```python
from build123d import *

# Parameters (mm, degrees)
AUFSATZ_LINEAR_AUSTRAGEN1_DEPTH      = 2.5
AUFSATZ_LINEAR_AUSTRAGEN1_DEPTH_BACK = 2.5
SKIZZE1_W                            = 100
SKIZZE1_H                            = 40
SCHNITT_LINEAR_AUSTRAGEN1_DEPTH      = 54.909646632
SCHNITT_LINEAR_AUSTRAGEN1_DEPTH_BACK = 54.909646632
SKIZZE2_R                            = 1.5
SCHNITT_LINEAR_AUSTRAGEN2_DEPTH      = 54.909646632
SCHNITT_LINEAR_AUSTRAGEN2_DEPTH_BACK = 54.909646632
SKIZZE7_W                            = 70
SKIZZE7_H                            = 40
AUFSATZ_LINEAR_AUSTRAGEN3_DEPTH      = 5
FASE1_SIZE                           = 2
SCHNITT_LINEAR_AUSTRAGEN7_DEPTH      = 55.371407927
SCHNITT_LINEAR_AUSTRAGEN7_DEPTH_BACK = 55.371407927
VERRUNDUNG1_R                        = 2
SCHNITT_LINEAR_AUSTRAGEN6_DEPTH      = 8.5
VERRUNDUNG2_R                        = 2
SCHNITT_LINEAR_AUSTRAGEN8_DEPTH      = 59.285933123
VERRUNDUNG3_R                        = 1
VERRUNDUNG4_R                        = 6


with BuildPart() as part:
    # Skizze1 → Aufsatz-Linear austragen1 (new, two sides: drawn at the far end of the back side and taken through both)
    with BuildSketch(Plane.XY.offset(-AUFSATZ_LINEAR_AUSTRAGEN1_DEPTH_BACK)):
        Rectangle(SKIZZE1_W, SKIZZE1_H)
    extrude(amount=AUFSATZ_LINEAR_AUSTRAGEN1_DEPTH + AUFSATZ_LINEAR_AUSTRAGEN1_DEPTH_BACK)

    # Skizze2 → Schnitt-Linear austragen1 (cut, two sides: drawn at the far end of the back side and taken through both)
    with BuildSketch(Plane.XY.offset(-SCHNITT_LINEAR_AUSTRAGEN1_DEPTH_BACK)):
        with Locations((-45, 15)):
            Circle(SKIZZE2_R)
        with Locations(Location((-45, -15, 0), (0, 0, 180))):
            Circle(SKIZZE2_R)
        with Locations((45, -15)):
            Circle(SKIZZE2_R)
        with Locations(Location((45, 15, 0), (0, 0, 180))):
            Circle(SKIZZE2_R)
    extrude(amount=SCHNITT_LINEAR_AUSTRAGEN1_DEPTH + SCHNITT_LINEAR_AUSTRAGEN1_DEPTH_BACK, mode=Mode.SUBTRACT)

    # Skizze4 → Schnitt-Linear austragen2 (cut, two sides: drawn at the far end of the back side and taken through both)
    with BuildSketch(Plane.XY.offset(-SCHNITT_LINEAR_AUSTRAGEN2_DEPTH_BACK)):
        with BuildLine():
            Line((-48, -8), (-48, 8))
            ThreePointArc((-48, 8), (-47.121320344, 10.121320344), (-45, 11))
            Line((-45, 11), (-40.5, 11))
            ThreePointArc((-40.5, 11), (-38.378679656, 10.121320344), (-37.5, 8))
            Line((-37.5, 8), (-37.5, -8))
            ThreePointArc((-37.5, -8), (-38.378679656, -10.121320344), (-40.5, -11))
            Line((-40.5, -11), (-45, -11))
            ThreePointArc((-45, -11), (-47.121320344, -10.121320344), (-48, -8))
        make_face()
        with BuildLine():
            Line((45, -11), (40.5, -11))
            ThreePointArc((40.5, -11), (38.378679656, -10.121320344), (37.5, -8))
            Line((37.5, -8), (37.5, 8))
            ThreePointArc((37.5, 8), (38.378679656, 10.121320344), (40.5, 11))
            Line((40.5, 11), (45, 11))
            ThreePointArc((45, 11), (47.121320344, 10.121320344), (48, 8))
            Line((48, 8), (48, -8))
            ThreePointArc((48, -8), (47.121320344, -10.121320344), (45, -11))
        make_face()
    extrude(amount=SCHNITT_LINEAR_AUSTRAGEN2_DEPTH + SCHNITT_LINEAR_AUSTRAGEN2_DEPTH_BACK, mode=Mode.SUBTRACT)

    # Skizze7 → Aufsatz-Linear austragen3 (add)
    with BuildSketch(Plane(origin=(0, 0, -2.5), x_dir=(-1, 0, 0), z_dir=(0, 0, -1))):
        Rectangle(SKIZZE7_W, SKIZZE7_H)
    extrude(amount=AUFSATZ_LINEAR_AUSTRAGEN3_DEPTH)

    # Fase1
    fase1_edges = [part.edges().sort_by_distance(p)[0] for p in [
        (50, 20, 0),
        (50, -20, 0),
        (-50, -20, 0),
        (-50, 20, 0),
    ]]
    chamfer(fase1_edges, length=FASE1_SIZE)

    # Skizze9 → Schnitt-Linear austragen7 (cut, two sides: drawn at the far end of the back side and taken through both)
    with BuildSketch(Plane.XY.offset(-SCHNITT_LINEAR_AUSTRAGEN7_DEPTH_BACK)):
        with BuildLine():
            Line((-3.5, -20), (3.5, -20))
            Line((3.5, -20), (3.5, -7))
            ThreePointArc((3.5, -7), (0, -3.5), (-3.5, -7))
            Line((-3.5, -7), (-3.5, -20))
        make_face()
    extrude(amount=SCHNITT_LINEAR_AUSTRAGEN7_DEPTH + SCHNITT_LINEAR_AUSTRAGEN7_DEPTH_BACK, mode=Mode.SUBTRACT)

    # Verrundung1
    verrundung1_edges = [part.edges().sort_by_distance(p)[0] for p in [
        (3.5, -20, -2.5),
        (-3.5, -20, -2.5),
    ]]
    fillet(verrundung1_edges, radius=VERRUNDUNG1_R)

    # Skizze8 → Schnitt-Linear austragen6 (cut)
    with BuildSketch(Plane.XY.offset(2.5)):
        with BuildLine():
            Line((6.5, -18), (30, -18))
            ThreePointArc((30, -18), (32.121320344, -17.121320344), (33, -15))
            Line((33, -15), (33, 15))
            ThreePointArc((33, 15), (32.121320344, 17.121320344), (30, 18))
            Line((30, 18), (-30, 18))
            ThreePointArc((-30, 18), (-32.121320344, 17.121320344), (-33, 15))
            Line((-33, 15), (-33, -15))
            ThreePointArc((-33, -15), (-32.121320344, -17.121320344), (-30, -18))
            Line((-30, -18), (-6.5, -18))
            ThreePointArc((-6.5, -18), (-5.792893219, -17.707106781), (-5.5, -17))
            Line((-5.5, -17), (-5.5, -7))
            ThreePointArc((-5.5, -7), (0, -1.5), (5.5, -7))
            Line((5.5, -7), (5.5, -17))
            ThreePointArc((5.5, -17), (5.792893219, -17.707106781), (6.5, -18))
        make_face()
    extrude(amount=-SCHNITT_LINEAR_AUSTRAGEN6_DEPTH, mode=Mode.SUBTRACT)

    # Verrundung2
    # the kernel refuses this fillet: 2 mm, written as the material it takes off along each edge
    with BuildSketch(Plane(origin=(-3.5, -7, -7.5), x_dir=(0, 0, 1), z_dir=(0, -1, 0)), Plane(origin=(3.5, -23, -7.5), x_dir=(0, 0, 1), z_dir=(0, 1, 0))) as verrundung2_piece_1:
        with BuildLine():
            CenterArc((VERRUNDUNG2_R, VERRUNDUNG2_R), VERRUNDUNG2_R, 180, 90)
            Line((0, VERRUNDUNG2_R), (0, 0))
            Line((0, 0), (VERRUNDUNG2_R, 0))
        make_face()
    extrude(amount=16, mode=Mode.SUBTRACT)
    with BuildSketch(Plane(origin=(0, -7, -7.5), x_dir=(-1, 0, 0), z_dir=(0, -1, 0))) as verrundung2_piece_2:
        with BuildLine():
            CenterArc((3.5 + VERRUNDUNG2_R, -VERRUNDUNG2_R), VERRUNDUNG2_R, 90, 90)
            Line((3.5 + VERRUNDUNG2_R, 0), (3.5, 0))
            Line((3.5, 0), (3.5, -VERRUNDUNG2_R))
        make_face()
    revolve(axis=Axis((0, -7, -7.5), (0, 0, -1)), revolution_arc=180, mode=Mode.SUBTRACT)

    # Skizze10 → Schnitt-Linear austragen8 (cut, through all)
    with BuildSketch(Plane(origin=(0, -9, 0), x_dir=(1, 0, 0), z_dir=(0, 1, 0))):
        Polygon((12, -2.5), (5.5, 4), (-5.5, 4), (-12, -2.5), align=None)
    extrude(amount=-SCHNITT_LINEAR_AUSTRAGEN8_DEPTH, mode=Mode.SUBTRACT)

    # Verrundung3
    verrundung3_edges = [part.edges().sort_by_distance(p)[0] for p in [
        (4.5, -9, 2.5),
        (4.5, -9, -4),
        (-4.5, -9, -4),
        (-4.5, -9, 2.5),
    ]]
    fillet(verrundung3_edges, radius=VERRUNDUNG3_R)

    # Verrundung4
    verrundung4_edges = [part.edges().sort_by_distance(p)[0] for p in [
        (12, -19, 2.5),
        (-12, -19, 2.5),
    ]]
    fillet(verrundung4_edges, radius=VERRUNDUNG4_R)


solid = part.part
```
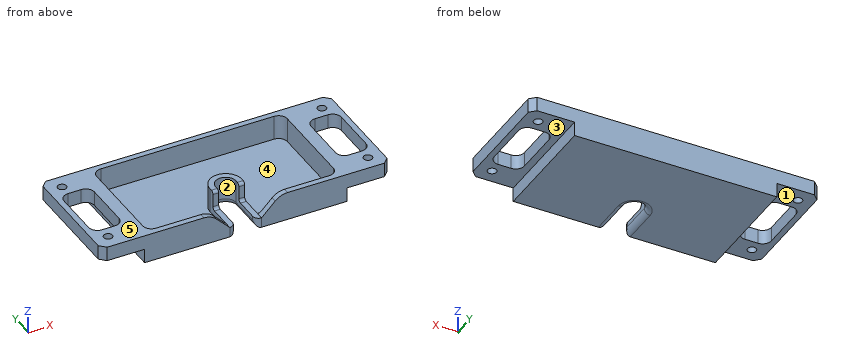
Geometry: final body of the model. Coordinates: model frame, mm. Face numbers are marked on the shaded views. A direction names the side the tool comes from. Coordinates: 2 decimals unless noted, no trailing zeros. Loops run counter-clockwise (first coordinate to the right, second up) from the corner with the lowest first, then second, coordinate; pieces in that order, holes last. Notation, with made-up numbers: (5.25, 23.25) -> (18.25, 23.25) arc R23 cw to (18.25, 31.25) -> close; hole circle Ø7 at (64, -10.5). An arc over 180 degrees is marked (long way). Use a Markdown table: item, result. Add a question column.
(1) Section query D-D, the plane x = 13.5. Return loops of the section in (y, z).
(2) Pin query (flat end, axial travel): pin 1 Ø2 at (x, z) = (-4.5, -0.5) entering from -Y; pin 2 Ø2 at (x, y) = (4, 9) entering from +Z; pin 3 Ø2.5 at (y, z) = (-5, -4.5) entering from -X. Return the tip coordinate at first contact, or that it passes through.
(3) Mould query, pull axis X, two halves, no side actions, for the marked faces 1 and 2. Classes: pulls with the +X half, pulls with the -X half, needs draft (parallel to the pull), parting line crosses it, or undercut.
(4) Access query for the marked faces 3, 4 and 5. Directions: +Z, -Z, +X, -X, +Y, -Y. A direction counts if a zero-diameter tool reaches every point of the face in a straight line with its end or side. Return the directions, or none.
(5) Section query C-C, the plane x = 0. Return loops of the section in (y, z).
(6) Section query A-A, the plane x = -22. Return loops of the section in (y, z), plus the area to 3 significant figures.
(7) Line query: line 1 along Y through (x, z) = (-45, 1.25); line 2 along X through (y, z) = (5.5, -1.75); line 3 along X through (y, z) = (-6.5, -3). Output: solid intervals per line, ascending.
(8) Section query B-B, the plane y = -5. State how many separate pieces and enclosed holes the cut face has, plus the area to 3 significant figures.
Answer:
| question | item | result |
|---|---|---|
| 1 | outline | (-20, -7.5) -> (20, -7.5) -> (20, 2.5) -> (18, 2.5) -> (18, -6) -> (-18, -6) -> (-18, 2.42) -> (-20, 2.42) -> close |
| 2 | pin 1 | stops at y = -9 |
| 2 | pin 2 | stops at z = -6 |
| 2 | pin 3 | stops at x = -35 |
| 3 | face 1 | needs draft |
| 3 | face 2 | undercut |
| 4 | face 3 | -Z, +X, +Y, -Y |
| 4 | face 4 | +Z |
| 4 | face 5 | +Z, +X, -X, +Y, -Y |
| 5 | outline | (-3.5, -5.5) arc R2 ccw to (-1.5, -7.5) -> (20, -7.5) -> (20, 2.5) -> (18, 2.5) -> (18, -6) -> (-1.5, -6) -> (-1.5, 2.5) -> (-3.5, 2.5) -> close |
| 6 | outline | (-20, -7.5) -> (20, -7.5) -> (20, 2.5) -> (18, 2.5) -> (18, -6) -> (-18, -6) -> (-18, 2.5) -> (-20, 2.5) -> close |
| 6 | area | 94.0 mm^2 |
| 7 | line 1 | y = -20 to -16.5, -13.5 to -11, 11 to 13.5, 16.5 to 20 |
| 7 | line 2 | x = -50 to -48, -37.5 to -33, 33 to 37.5, 48 to 50 |
| 7 | line 3 | x = -35 to -33, -5.48 to -3.46, 3.46 to 5.48, 33 to 35 |
| 8 | separate pieces | 4 |
| 8 | enclosed holes | 0 |
| 8 | area | 212 mm^2 |
